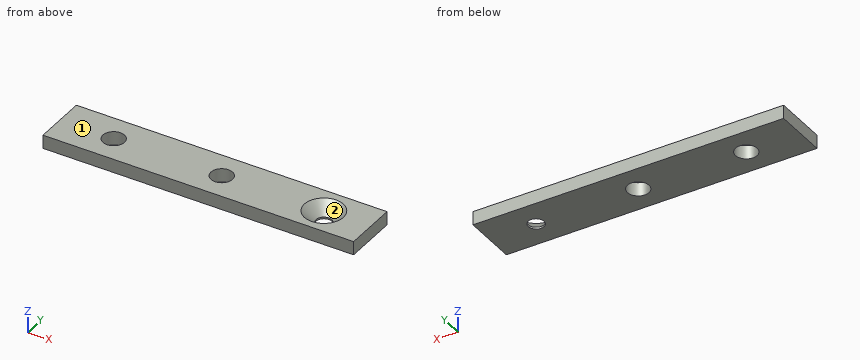
```python
from build123d import *

# Parameters (mm, degrees)
SKETCH1_R           = 2.54
BOSS_EXTRUDE1_DEPTH = 3.175
SKETCH3_R           = 1.5875
CUT_EXTRUDE1_DEPTH  = 49.15125907
CUT_EXTRUDE1_DRAFT  = 5
CHAMFER1_SIZE       = 3
CHAMFER1_SIZE2      = 2.769187039


with BuildPart() as part:
    # Sketch1 → Boss-Extrude1 (new body)
    with BuildSketch(Plane.XY):
        Polygon((47.625, 6.35), (47.625, -6.35), (25.4, -6.35), (-25.4, -6.35), (-25.4, 6.35), (25.4, 6.35), align=None)
        with Locations((12.7, 0)):
            Circle(SKETCH1_R, mode=Mode.SUBTRACT)
        with Locations((-12.7, 0)):
            Circle(SKETCH1_R, mode=Mode.SUBTRACT)
    extrude(amount=BOSS_EXTRUDE1_DEPTH)


with BuildPart() as cut_extrude1_tool:
    # Sketch3 → Cut-Extrude1 (with draft: the straight prism first)
    with BuildSketch(Plane.XY.offset(3.175)):
        with Locations((36.703, 0)):
            Circle(SKETCH3_R)
    extrude(amount=-CUT_EXTRUDE1_DEPTH)
    # Cut-Extrude1: the draft: its side faces are tilted about the plane it starts from
    cut_extrude1_sides = [cut_extrude1_tool.faces().sort_by_distance(p)[0] for p in [
        (35.1155, 0, -21.400629535),
    ]]
    draft(cut_extrude1_sides, Plane.XY.offset(3.175), CUT_EXTRUDE1_DRAFT)


with BuildPart() as part_1:
    add(part.part)

    # Cut-Extrude1: cut by cut_extrude1_tool
    add(cut_extrude1_tool.part, mode=Mode.SUBTRACT)

    # Chamfer1
    chamfer1_edges = [part_1.edges().sort_by_distance(p)[0] for p in [
        (35.1155, 0, 3.175),
    ]]
    chamfer1_side = [part_1.faces().sort_by_distance(p)[0] for p in [
        (46.883788787, 0, 3.175),
    ]]
    chamfer(chamfer1_edges, length=CHAMFER1_SIZE, length2=CHAMFER1_SIZE2, reference=chamfer1_side[0])


solid = part_1.part
```
Verification items for the finished model (mm, model axes). Face numbers are marked on the shaded views. Coordinates: 2 decimals unless noted, no trailing zeros. Order: outer loops, then holes, each group sorted by start corner. A loop starts at its lowest first (then second) coordinate and runs counter-clockwise, first axis right, second up. Notation, with made-up numbers: (-19, 58.25) -> (16, 58.25) arc R15 cw to (16, 87.25) -> close; hole circle Ø1 at (7, 41.5). An arc over 180 degrees is marked (long way). Answer as CSV lines item,"result". Start each with the question number.
1) Cross-section at B-B, the plane y = 0. Record the boundary of the cut face in (x, z) (1 decimal).
2) Cross-section at A-A, the plane x = -12.7. Record the boundary of the cut face in (y, z) (3 decimals).
3) Material ranges on L1, parallel to Y at x = -12.7, z = 2.15; L2, parallel to X at y = -0.75, z = 1.1 (3 decimals); L3, parallel to X at y = 1.5, z = 2 (3 decimals), recorded low to high. Write a range as [from, to].
4) Cross-section at D-D, the plane x = 14.5. Record the boundary of the cut face in (y, z) (3 decimals), then the cut area to 3 significant figures.
5) Cross-section at C-C, the plane z = 2.15. Give the number of separate pieces and of enclosed holes in the cut face, then the cut area to 3 significant figures.
6) Release check for a two-part mould opening along Y. For the marked faces 1 and 2 record: released by +Y, released by -Y, zero draft, split by the parting line, or undercut.
Conclusion:
1,outline,"(-25.4, 0) -> (-15.2, 0) -> (-15.2, 3.2) -> (-25.4, 3.2) -> close; (-10.2, 0) -> (10.2, 0) -> (10.2, 3.2) -> (-10.2, 3.2) -> close; (15.2, 0) -> (34.8, 0) -> (34.9, 0.4) -> (32.1, 3.2) -> (15.2, 3.2) -> close; (38.5, 0.4) -> (38.6, 0) -> (47.6, 0) -> (47.6, 3.2) -> (41.3, 3.2) -> close"
2,outline,"(-6.35, 0) -> (-2.54, 0) -> (-2.54, 3.175) -> (-6.35, 3.175) -> close; (2.54, 0) -> (6.35, 0) -> (6.35, 3.175) -> (2.54, 3.175) -> close"
3,L1,"y = [-6.35, -2.54], [2.54, 6.35]"
3,L2,"x = [-25.4, -15.127], [-10.273, 10.273], [15.127, 34.305], [39.101, 47.625]"
3,L3,"x = [-25.4, -14.75], [-10.65, 10.65], [14.75, 33.638], [39.768, 47.625]"
4,outline,"(-6.35, 0) -> (-1.792, 0) -> (-1.792, 3.175) -> (-6.35, 3.175) -> close; (1.792, 0) -> (6.35, 0) -> (6.35, 3.175) -> (1.792, 3.175) -> close"
4,area,"28.9 mm²"
5,separate pieces,"1"
5,enclosed holes,"3"
5,area,"847 mm²"
6,face 1,"zero draft"
6,face 2,"undercut"
